Source: CAD feature listing. Evaluate the final solid. Frame: model axes, mm. Face numbers are marked on the shaded views. A direction names the side the tool comes from. Give positions to 0.01 mm unless a question says otherwise; leave off trailing zeros. Order: outer loops, then holes, each group sorted by start corner. A loop starts at its lowest first (then second) coordinate and runs counter-clockwise, first axis right, second up. Notation, with made-up numbers: (84, 24) -> (105, 24) arc R14 ccw to (105, 46) -> close; hole circle Ø5 at (65.5, -7). An arc over 180 degrees is marked (long way). Answer in a Markdown table with one row per item.
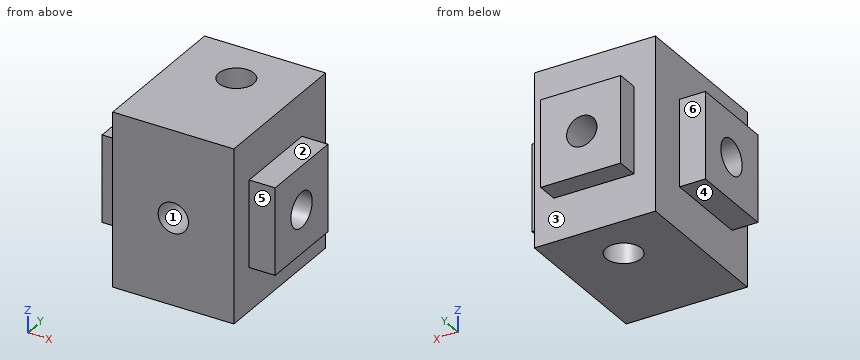
```python
from build123d import *

# Parameters (mm, degrees)
F0_W      = 40
F0_H      = 40
F1_DEPTH  = 40
F2_R      = 4.05
F3_DEPTH  = 40
F4_R      = 4.05
F5_DEPTH  = 40
F6_R      = 3.5
F7_DEPTH  = 40
F8_W      = 40
F8_H      = 40
F8_W_2    = 20.1
F8_H_2    = 20
F9_DEPTH  = 6
F10_W     = 34
F10_H     = 40
F10_W_2   = 18.5
F10_H_2   = 20
F11_DEPTH = 5
F12_W     = 35
F12_H     = 40
F12_W_2   = 20
F12_H_2   = 20
F13_DEPTH = 6


with BuildPart() as f1:
    # F0 (on Top) → F1 (new body)
    with BuildSketch(Plane.XY):
        Rectangle(F0_W, F0_H)
    extrude(amount=F1_DEPTH)

    # F2 (on face) → F3 (cut)
    with BuildSketch(Plane.XY.offset(40)):
        with Locations((0, 4.0336288512)):
            Circle(F2_R)
    extrude(amount=-F3_DEPTH, mode=Mode.SUBTRACT)

    # F4 (on face) → F5 (cut)
    with BuildSketch(Plane.YZ.offset(20)):
        with Locations((-4.1, 20)):
            Circle(F4_R)
    extrude(amount=-F5_DEPTH, mode=Mode.SUBTRACT)

    # F6 (on face) → F7 (cut)
    with BuildSketch(Plane(origin=(0, 20, 0), x_dir=(-1, 0, 0), z_dir=(0, 1, 0))):
        with Locations((0, 20)):
            Circle(F6_R)
    extrude(amount=-F7_DEPTH, mode=Mode.SUBTRACT)

    # F8 (on face) → F9 (cut)
    with BuildSketch(Plane.YZ.offset(20)):
        with Locations((0, 20)):
            Rectangle(F8_W, F8_H)
        with Locations((-4.1, 20)):
            Rectangle(F8_W_2, F8_H_2, mode=Mode.SUBTRACT)
    extrude(amount=-F9_DEPTH, mode=Mode.SUBTRACT)

    # F10 (on face) → F11 (cut)
    with BuildSketch(Plane(origin=(0, 20, 0), x_dir=(-1, 0, 0), z_dir=(0, 1, 0))):
        with Locations((3, 20)):
            Rectangle(F10_W, F10_H)
        with Locations((-0.25, 20)):
            Rectangle(F10_W_2, F10_H_2, mode=Mode.SUBTRACT)
    extrude(amount=-F11_DEPTH, mode=Mode.SUBTRACT)

    # F12 (on face) → F13 (cut)
    with BuildSketch(Plane(origin=(-20, 0, 0), x_dir=(0, -1, 0), z_dir=(-1, 0, 0))):
        with Locations((2.5, 20)):
            Rectangle(F12_W, F12_H)
        with Locations((4.15, 20.0738927722)):
            Rectangle(F12_W_2, F12_H_2, mode=Mode.SUBTRACT)
    extrude(amount=-F13_DEPTH, mode=Mode.SUBTRACT)


solid = f1.part
```
(1) First-contact query: pin 1 Ø1.8 at (x, y) = (-16.5, -8.5) entering from -Z; pin 2 Ø1.8 at (x, z) = (-16.5, 24) entering from -Y; pin 3 Ø3 at (x, y) = (17.5, -5.5) entering from +Z. Flat tips, straight axial feed; report the tip coordinate or a pass-through.
A:
| item | result |
|---|---|
| pin 1 | stops at z = 10.07 |
| pin 2 | stops at y = -14.15 |
| pin 3 | stops at z = 30 |
(2) Ray query, probe 1 along X at (y, z) = (1, 20); probe 2 along Y at (x, z) = (9, 16.5); probe 3 along X at (y, z) = (-9.5, 34.5). Return the intervals inside material, ascending.
A:
| item | result |
|---|---|
| probe 1 | x = -20 to -3.5, 3.5 to 20 |
| probe 2 | y = -20 to -6.14, -2.06 to 20 |
| probe 3 | x = -14 to 14 |
(3) Pull-direction query (Z, two-part tool) for the marked faces 1, 2 and 3; classes: +Z half, -Z half, draft (parallel to the pull), parting line (faces both ways), or undercut.
A:
| item | result |
|---|---|
| face 1 | undercut |
| face 2 | +Z half |
| face 3 | draft |
(4) Section query B-B (x = 0). Return the cut outline in (y, z), plus the area to 3 significant figures.
A:
| item | result |
|---|---|
| outline | (-20, 0) -> (-0.02, 0) -> (-0.02, 16.5) -> (-2.06, 16.5) arc R4.05 cw to (-6.14, 16.5) -> (-20, 16.5) -> close; (-20, 23.5) -> (-6.14, 23.5) arc R4.05 cw to (-2.06, 23.5) -> (-0.02, 23.5) -> (-0.02, 40) -> (-20, 40) -> close; (8.08, 0) -> (15, 0) -> (15, 10) -> (20, 10) -> (20, 16.5) -> (8.08, 16.5) -> close; (8.08, 23.5) -> (20, 23.5) -> (20, 30) -> (15, 30) -> (15, 40) -> (8.08, 40) -> close |
| area | 950 mm^2 |
(5) Section query A-A (y = -4.1). Return the cut outline in (x, z).
A:
| item | result |
|---|---|
| outline | (-20, 10.07) -> (-14, 10.07) -> (-14, 0) -> (14, 0) -> (14, 10) -> (20, 10) -> (20, 15.95) -> (-20, 15.95) -> close; (-20, 24.05) -> (20, 24.05) -> (20, 30) -> (14, 30) -> (14, 40) -> (-14, 40) -> (-14, 30.07) -> (-20, 30.07) -> close |
(6) Section query C-C (z = 22). Give the number of separate pieces and of enclosed holes in the cut face, plus the area to 3 significant figures.
A:
| item | result |
|---|---|
| separate pieces | 4 |
| enclosed holes | 0 |
| area | 833 mm^2 |
(7) Access query for the marked faces 4, 5 and 6. Directions: +Z, -Z, +X, -X, +Y, -Y. A direction counts if a zero-diameter tool reaches every point of the face in a straight line with its end or side. Return the directions, or none.
A:
| item | result |
|---|---|
| face 4 | -Z, -X, +Y, -Y |
| face 5 | +Z, -Z, +X, -Y |
| face 6 | +Z, -Z, -X, +Y |
(8) Section query D-D (x = 5). Return the cut outline in (y, z).
A:
| item | result |
|---|---|
| outline | (-20, 0) -> (15, 0) -> (15, 10) -> (20, 10) -> (20, 30) -> (15, 30) -> (15, 40) -> (-20, 40) -> close; hole circle Ø8.1 at (-4.1, 20) |
